Part model, mm, in its own coordinate system. A direction names the side the tool comes from. Give positions to 0.01 mm unless a question says otherwise; leave off trailing zeros. Write each loop counter-clockwise with the first axis right and the second up, starting at its lowest first coordinate (ties: lowest second). Pieces come first, ordered by that corner, then holes. Notation, with made-up numbers: (20, 88) - (77, 88) arc R17 cw to (77, 115) - close; hole circle Ø7 at (-6.5, 66). An arc over 180 degrees is marked (long way). Answer in a Markdown table with one row per item. Add a question column.
1. Which spindle directions (+Z, -Z, +X, -X, +Y, -Y) get a long thin tool onto all of the face, cutting with end or side? Do faces 1 (the flat face through (-29, 88.083, -12)), 2 (the flat face through (-29, 89.033, 0)), 3 (the flat face through (-29, 93.533, 0)). Say none if no direction does.
2. Band-saw the part on A-A on y = 88.5. Write the cut outline in (x, z).
3. Band-saw the part on D-D on z = 2.75. Write the cut outline in (x, y), plus the area to 4 significant figures.
4. Band-saw the part on C-C on y = 91.5. Write the cut outline in (x, z), plus the area to 3 significant figures.
5. Drop flat-ended pins along their axis: pin 1 Ø3 at (x, y) = (-29, 94.5) entering from +Z; pin 2 Ø1.3 at (y, z) = (91.5, -1.5) entering from +X; pin 3 Ø2 at (y, z) = (92, -2) entering from -X. Give the stop position or say it passes through.
6. Band-saw the part on B-B on x = -28. Write the cut outline in (y, z).
7. Probe line 1 along X through (y, z) = (91.25, -11.5); line 2 along Y through (x, z) = (-30.75, -12.5); line 3 along X through (y, z) = (90.75, -2.5). List the from-to ranges inside material, lowest first.
8. Pull direction X, two halves, no side cores. Call faces 4 (the flat face through (-26.203, 91, 0)), 5 (the flat face through (-29, 94.483, -12)), 6 (the flat face through (-30.8, 91.3, 5.1)), 7 (the flat face through (-26, 91, -5.4)): released by +X, released by -X, zero draft, split by the parting line, or undercut.
```python
from build123d import *

# Parameters (mm, degrees)
SKETCH2_W                = 8.799999809
SKETCH2_H                = 8.79999981
SKETCH2_W_2              = 6.399999809
SKETCH2_H_2              = 6.39999981
BOSS_EXTRUDE1_DEPTH      = 2
BOSS_EXTRUDE1_DEPTH_BACK = 2
SKETCH3_W                = 8.799999809
SKETCH3_H                = 8.79999981
BOSS_EXTRUDE2_DEPTH      = 5
SKETCH4_W                = 5.099999879
SKETCH4_H                = 4.499999898
BOSS_EXTRUDE3_DEPTH      = 11
CHAMFER1_SIZE            = 1


with BuildPart() as part:
    # Sketch2 → Boss-Extrude1 (new body, two sides)
    with BuildSketch(Plane.XY.offset(-12.400000378)) as boss_extrude1_sk:
        with Locations((-28.752555167, 91.282627708)):
            Rectangle(SKETCH2_W, SKETCH2_H)
        with Locations((-28.752555167, 91.282627708)):
            Rectangle(SKETCH2_W_2, SKETCH2_H_2, mode=Mode.SUBTRACT)
    extrude(amount=BOSS_EXTRUDE1_DEPTH)
    extrude(boss_extrude1_sk.sketch, amount=-BOSS_EXTRUDE1_DEPTH_BACK)

    # Sketch3 → Boss-Extrude2 (add)
    with BuildSketch(Plane.XY.offset(-10.400000378)):
        with Locations((-28.752555167, 91.282627708)):
            Rectangle(SKETCH3_W, SKETCH3_H)
    extrude(amount=BOSS_EXTRUDE2_DEPTH)

    # Sketch4 → Boss-Extrude3 (add)
    with BuildSketch(Plane.XY.offset(-5.400000378)):
        with Locations((-28.752555167, 91.282627708)):
            Rectangle(SKETCH4_W, SKETCH4_H)
    extrude(amount=BOSS_EXTRUDE3_DEPTH)

    # Chamfer1
    chamfer1_edges = [part.edges().sort_by_distance(p)[0] for p in [
        (-31.302555106, 91.282627708, 5.599999622),
        (-28.752555166, 89.032627759, 5.599999622),
        (-26.202555227, 91.282627708, 5.599999622),
        (-28.752555166, 93.532627657, 5.599999622),
    ]]
    chamfer(chamfer1_edges, length=CHAMFER1_SIZE)


solid = part.part
```
Values:
| question | item | result |
|---|---|---|
| 1 | face 1 | -Z |
| 1 | face 2 | +Z, +X, -X, -Y |
| 1 | face 3 | +Z, +X, -X, +Y |
| 2 | outline | (-33.15, -14.4) - (-31.95, -14.4) - (-31.95, -10.4) - (-25.55, -10.4) - (-25.55, -14.4) - (-24.35, -14.4) - (-24.35, -5.4) - (-33.15, -5.4) - close |
| 3 | outline | (-31.3, 89.03) - (-26.2, 89.03) - (-26.2, 93.53) - (-31.3, 93.53) - close |
| 3 | area | 22.95 mm² |
| 4 | outline | (-33.15, -14.4) - (-31.95, -14.4) - (-31.95, -10.4) - (-25.55, -10.4) - (-25.55, -14.4) - (-24.35, -14.4) - (-24.35, -5.4) - (-26.2, -5.4) - (-26.2, 4.6) - (-27.2, 5.6) - (-30.3, 5.6) - (-31.3, 4.6) - (-31.3, -5.4) - (-33.15, -5.4) - close |
| 4 | area | 109 mm² |
| 5 | pin 1 | stops at z = 5.13 |
| 5 | pin 2 | stops at x = -26.2 |
| 5 | pin 3 | stops at x = -31.3 |
| 6 | outline | (86.88, -14.4) - (88.08, -14.4) - (88.08, -10.4) - (94.48, -10.4) - (94.48, -14.4) - (95.68, -14.4) - (95.68, -5.4) - (93.53, -5.4) - (93.53, 4.6) - (92.53, 5.6) - (90.03, 5.6) - (89.03, 4.6) - (89.03, -5.4) - (86.88, -5.4) - close |
| 7 | line 1 | x = -33.15 to -31.95, -25.55 to -24.35 |
| 7 | line 2 | y = 86.88 to 88.08, 94.48 to 95.68 |
| 7 | line 3 | x = -31.3 to -26.2 |
| 8 | face 4 | released by +X |
| 8 | face 5 | undercut |
| 8 | face 6 | released by -X |
| 8 | face 7 | zero draft |
